```python
from build123d import *

# Parameters (mm, degrees)
SKETCH_1_W      = 15
SKETCH_1_H      = 42
SKETCH_1_R      = 1.6
SKETCH_1_W_2    = 5
EXTRUDE_1_DEPTH = 6


with BuildPart() as part:
    # 草图1 → 凸台-拉伸1 (new body)
    # profile 1 of 7: a face of its own
    with BuildSketch(Plane.XY):
        with BuildLine():
            Line((0, 14), (0, 21))
            ThreePointArc((0, 21), (-21, 0), (0, -21))
            Line((0, -21), (0, -14))
            ThreePointArc((0, -14), (-1.471960144, -13.354006401), (-1.993043457, -11.833333333))
            ThreePointArc((-1.993043457, -11.833333333), (-8.485281374, -8.485281374), (-11.833333333, -1.993043457))
            ThreePointArc((-11.833333333, -1.993043457), (-14, 0), (-11.833333333, 1.993043457))
            ThreePointArc((-11.833333333, 1.993043457), (-8.485281374, 8.485281374), (-1.993043457, 11.833333333))
            ThreePointArc((-1.993043457, 11.833333333), (-1.471960144, 13.354006401), (0, 14))
        make_face()
    # profile 2 of 7: a face of its own
    with BuildSketch(Plane.XY):
        with BuildLine():
            ThreePointArc((0, 10), (-1.354006401, 10.528039856), (-1.993043457, 11.833333333))
            ThreePointArc((-1.993043457, 11.833333333), (-8.485281374, 8.485281374), (-11.833333333, 1.993043457))
            ThreePointArc((-11.833333333, 1.993043457), (-10.528039856, 1.354006401), (-10, 0))
            ThreePointArc((-10, 0), (-10.528039856, -1.354006401), (-11.833333333, -1.993043457))
            ThreePointArc((-11.833333333, -1.993043457), (-8.485281374, -8.485281374), (-1.993043457, -11.833333333))
            ThreePointArc((-1.993043457, -11.833333333), (-1.354006401, -10.528039856), (0, -10))
            Line((0, -10), (0, 10))
        make_face()
    # profile 3 of 7: a face of its own
    with BuildSketch(Plane.XY):
        with BuildLine():
            ThreePointArc((1.993043457, 11.833333333), (1.354006401, 10.528039856), (0, 10))
            Line((0, 10), (0, -10))
            ThreePointArc((0, -10), (1.354006401, -10.528039856), (1.993043457, -11.833333333))
            ThreePointArc((1.993043457, -11.833333333), (8.485281374, -8.485281374), (11.833333333, -1.993043457))
            ThreePointArc((11.833333333, -1.993043457), (10, 0), (11.833333333, 1.993043457))
            ThreePointArc((11.833333333, 1.993043457), (8.485281374, 8.485281374), (1.993043457, 11.833333333))
        make_face()
    # profile 4 of 7: a face of its own
    with BuildSketch(Plane.XY):
        with BuildLine():
            ThreePointArc((21, 0), (14.849242405, 14.849242405), (0, 21))
            Line((0, 21), (0, 14))
            ThreePointArc((0, 14), (1.414213562, 13.414213562), (2, 12))
            ThreePointArc((2, 12), (1.998260107, 11.916594108), (1.993043457, 11.833333333))
            ThreePointArc((1.993043457, 11.833333333), (8.485281374, 8.485281374), (11.833333333, 1.993043457))
            ThreePointArc((11.833333333, 1.993043457), (13.354006401, 1.471960144), (14, 0))
            ThreePointArc((14, 0), (13.354006401, -1.471960144), (11.833333333, -1.993043457))
            ThreePointArc((11.833333333, -1.993043457), (8.485281374, -8.485281374), (1.993043457, -11.833333333))
            ThreePointArc((1.993043457, -11.833333333), (1.998260107, -11.916594108), (2, -12))
            ThreePointArc((2, -12), (1.414213562, -13.414213562), (0, -14))
            Line((0, -14), (0, -21))
            ThreePointArc((0, -21), (14.849242405, -14.849242405), (21, 0))
        make_face()
    # profile 5 of 7: a face of its own
    with BuildSketch(Plane.XY):
        with BuildLine():
            Line((25, 21), (0, 21))
            ThreePointArc((0, 21), (14.849242405, 14.849242405), (21, 0))
            ThreePointArc((21, 0), (14.849242405, -14.849242405), (0, -21))
            Line((0, -21), (25, -21))
            Line((25, -21), (25, 21))
        make_face()
    # profile 6 of 7: a face of its own
    with BuildSketch(Plane.XY):
        with Locations((32.5, 0)):
            Rectangle(SKETCH_1_W, SKETCH_1_H)
        with Locations((32.4, 0)):
            Circle(SKETCH_1_R, mode=Mode.SUBTRACT)
        with Locations((29.5, -12)):
            Circle(SKETCH_1_R, mode=Mode.SUBTRACT)
        with Locations((35.5, -12)):
            Circle(SKETCH_1_R, mode=Mode.SUBTRACT)
        with Locations((35.5, 15)):
            Circle(SKETCH_1_R, mode=Mode.SUBTRACT)
        with Locations((29.5, 15)):
            Circle(SKETCH_1_R, mode=Mode.SUBTRACT)
    # profile 7 of 7: a face of its own
    with BuildSketch(Plane.XY):
        with Locations((42.5, 0)):
            Rectangle(SKETCH_1_W_2, SKETCH_1_H)
    extrude(amount=EXTRUDE_1_DEPTH)


solid = part.part
```
Check sheet for the modelled part. Datum: model origin and axes. Units: mm. Round coordinates to 2 decimals unless told otherwise and drop trailing zeros. Order: outer loops, then holes, each group sorted by start corner. A loop starts at its lowest first (then second) coordinate and runs counter-clockwise, first axis right, second up. Notation, with made-up numbers: (20.25, 45.25) -> (55.25, 45.25) arc R14 cw to (55.25, 51.25) -> close; hole circle Ø9 at (60.25, 50.25). An arc over 180 degrees is marked (long way). One line per item, written item: value. Start each with the question number.
Q1. Cross-section at C-C (y = 15). Record the boundary of the cut face in (x, z).
Q2. Gauge pin test, flat end, axial feed: pin 1 Ø2.5 at (x, y) = (35.5, 15) entering from +Z. Record the tip position at first contact, or that the pin passes through.
Q3. Mould release check, pull along Y, two halves, no side actions. Record for faces 1 (the face through (19, 0, 0)), 2 (the face through (34, 0, 3)), 3 (the face through (-21, 0, 3)): pulls with the +Y half, pulls with the -Y half, needs draft (parallel to the pull), parting line crosses it, or undercut.
Q4. Cross-section at A-A (x = 32.4). Record the boundary of the cut face in (y, z).
Q5. Cross-section at B-B (z = 2.35). Give the number of separate pieces and of enclosed holes in the cut face, and give its area (3 significant figures).
Q6. Cross-section at D-D (y = -15). Record the boundary of the cut face in (x, z), and give its area (3 significant figures).
Q7. Thickness scan on line 1 (Y direction, x = 35.5, z = 4.05); line 2 (Y direction, x = 34.5, z = 0.7); line 3 (Y direction, x = -12, z = 3.4). Record the ranges inside material, lowest first.
Completed:
1. outline: (-14.7, 0) -> (27.9, 0) -> (27.9, 6) -> (-14.7, 6) -> close; (31.1, 0) -> (33.9, 0) -> (33.9, 6) -> (31.1, 6) -> close; (37.1, 0) -> (45, 0) -> (45, 6) -> (37.1, 6) -> close
2. pin 1: passes through
3. face 1: needs draft
3. face 2: undercut
3. face 3: parting line crosses it
4. outline: (-21, 0) -> (-1.6, 0) -> (-1.6, 6) -> (-21, 6) -> close; (1.6, 0) -> (21, 0) -> (21, 6) -> (1.6, 6) -> close
5. separate pieces: 1
5. enclosed holes: 9
5. area: 2,490 mm²
6. outline: (-14.7, 0) -> (45, 0) -> (45, 6) -> (-14.7, 6) -> close
6. area: 358 mm²
7. line 1: y = -21 to -13.6, -10.4 to 13.4, 16.6 to 21
7. line 2: y = -21 to -13.25, -10.75 to 13.75, 16.25 to 21
7. line 3: y = -17.23 to -2, 2 to 17.23
